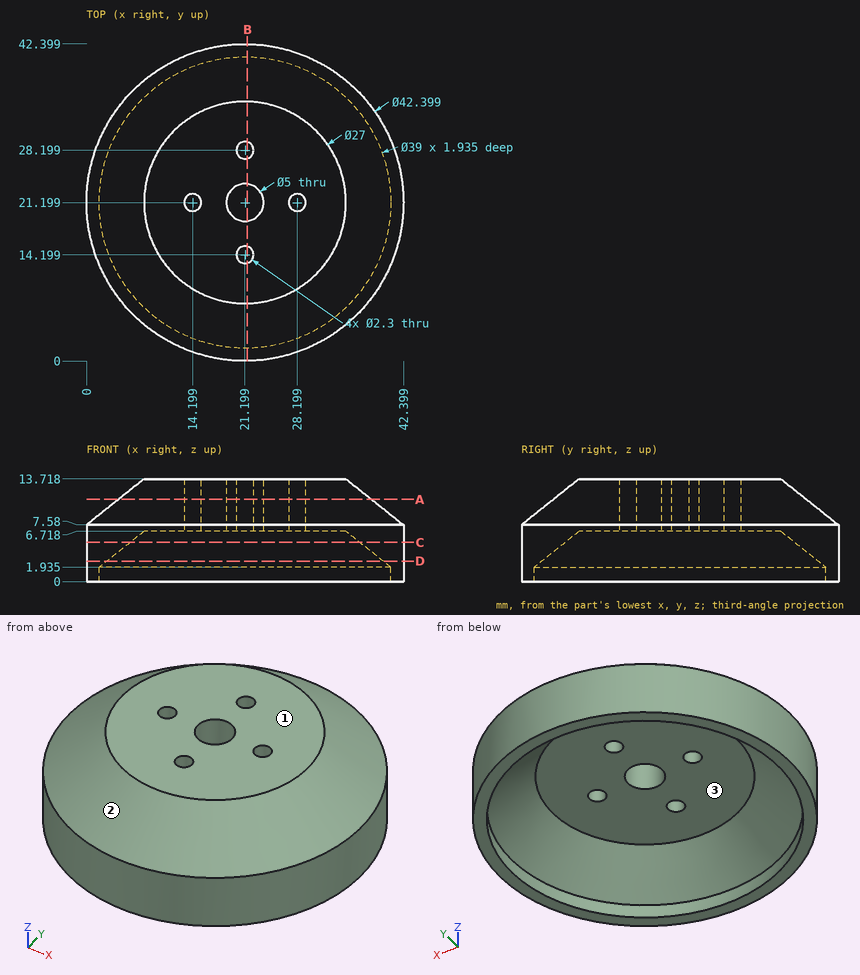
Study the drawing (mm; zero at the part's minimum x, y, z) and answer. Coordinates: 2 decimals unless noted, no trailing zeros. Loops run counter-clockwise (first coordinate to the right, second up) from the corner with the lowest first, then second, coordinate; pieces in that order, holes last. Notation, with made-up numbers: M 16,-28 L 75,-28 A26 ccw 75,5 Z; hole C -6.5,26.25 d11. An arc over 180 degrees is marked long. Answer in a Markdown table with one row per item.
1) Find section A-A (z = 11). Determine the outline of the cut face in (x, y).
Answers below:
| item | result |
|---|---|
| outline | C 21.2,21.2 d33.82; hole C 14.2,21.2 d2.3; hole C 21.2,21.2 d5; hole C 21.2,14.2 d2.3; hole C 21.2,28.2 d2.3; hole C 28.2,21.2 d2.3 |
2) Find section B-B (x = 21.5). Count the separate pieces of the cut face and the enclosed holes in it, then the cut area to 3 significant figures.
Answers below:
| item | result |
|---|---|
| separate pieces | 4 |
| enclosed holes | 0 |
| area | 235 mm^2 |
3) Find section D-D (z = 2.75). Determine the outline of the cut face in (x, y) (1 decimal).
Answers below:
| item | result |
|---|---|
| outline | C 21.2,21.2 d42.4; hole C 21.2,21.2 d37 |
4) Given pin 1 (6.5 mm diameter, centred on x = 21.2, y = 21.2, fed in from -Z); pin 2 (6 mm diameter, centred on y = 36, z = 11.5, fed in from -X) (1 decimal); pin 3 (3 mm diameter, centred on y = 4.5, z = 7.5, fed in from -X); pin 4 (1.8 mm diameter, centred on x = 21.2, y = 14.2, fed in from -Z), each flat-ended and moving along its own axis, determine where each tip first touches the part or whether it passes through.
Answers below:
| item | result |
|---|---|
| pin 1 | z = 6.72 |
| pin 2 | x = 6.9 |
| pin 3 | x = 6.42 |
| pin 4 | through |
5) Determine the mould class of the marked faces 1, 2 and 3 for opening direction Y: released by +Y, released by -Y, zero draft, split by the parting line, or undercut.
Answers below:
| item | result |
|---|---|
| face 1 | zero draft |
| face 2 | split by the parting line |
| face 3 | undercut |
6) Find section C-C (z = 5.25). Determine the outline of the cut face in (x, y).
Answers below:
| item | result |
|---|---|
| outline | C 21.2,21.2 d42.4; hole C 21.2,21.2 d30.68 |
7) Find the intervals of material crossed by probe 1 along Z at (x, y) = (19, 13.5); probe 2 along Y at (x, z) = (16.5, 4.75) (1 decimal); probe 3 along X at (y, z) = (31, 5) (1 decimal), in increasing order.
Answers below:
| item | result |
|---|---|
| probe 1 | 6.72 to 13.72 |
| probe 2 | 0.5 to 5.9, 36.5 to 41.9 |
| probe 3 | 2.4 to 9, 33.4 to 40 |
